Check sheet for the drawn part. Datum: minimum x, y, z corner. Units: mm. Give positions to 0.01 mm unless a question says otherwise; leave off trailing zeros.
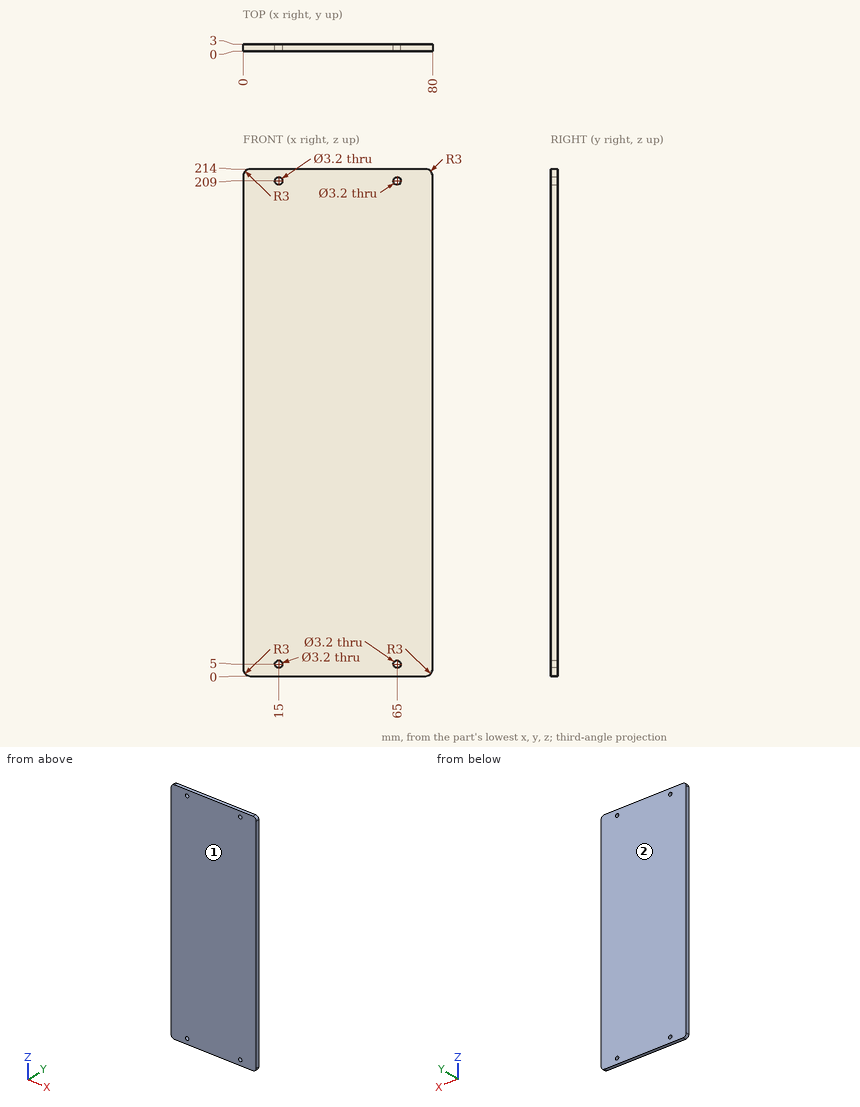
1) Draft check along Y on the marked faces 1 and 2. Enter one of: +Y half, -Y half, draft (parallel to the pull), parting line (faces both ways), or undercut.
2) Gauge pin test, flat ends, axial feed: pin 1 (5 mm diameter, centred on x = 65, z = 5, fed in from +Y); pin 2 (2.5 mm diameter, centred on x = 65, z = 209, fed in from -Y). Record the tip position at first contact, or that the pin passes through.
3) Scan lines: L1, parallel to X at y = 1.3, z = 5; L2, parallel to Z at x = 65, y = 0.85. Record each from-to range of solid material in increasing order.
Answers below:
1. face 1: -Y half
1. face 2: +Y half
2. pin 1: stops at y = 3
2. pin 2: passes through
3. L1: x = 0 to 13.4, 16.6 to 63.4, 66.6 to 80
3. L2: z = 0 to 3.4, 6.6 to 207.4, 210.6 to 214
